Work out the finished part from the listing and answer in its coordinate system (mm). Coordinates: 2 decimals unless noted, no trailing zeros. Order: outer loops, then holes, each group sorted by start corner. A loop starts at its lowest first (then second) coordinate and runs counter-clockwise, first axis right, second up. Notation, with made-up numbers: M 65,-31 L 78,-31 A12 ccw 78,-17 Z; hole C 54.5,15.5 d5. An arc over 180 degrees is marked long. Write item = value, one per line. Start each with the question number.
Q1. Determine the mould class of faces 1 (the cylindrical face through (-43.24, -3.81, 0.81)), 2 (the flat face through (-6, -34.374, 1)), 3 (the flat face through (35.7, -17, 1)) for opening direction Y: released by +Y, released by -Y, zero draft, split by the parting line, or undercut.
Q2. This flat-tipped pin is pushed along its axis until it touches: P1, Ø1.8, axis at x = -42.05, y = -2.9, coming from the +Z side. Where does it stop, or does it pass through?
Q3. Straight lines are drawn through the part: line 1 along Y through (x, z) = (31.65, 0.5); line 2 along Y through (x, z) = (-5.2, 0.6); line 3 along X through (y, z) = (-3.7, 1). For each, find the intervals that lie inside material, in ascending order.
Q4. Find section A-A on x = 31.65. Give the vertices of the cut face in (y, z), and give its area (3 significant figures).
Autodesk Inventor part; units mm, degrees
ref_plane "YZ Plane" through (0, 0, 0) normal (1, 0, 0) x (0, 1, 0)
ref_plane "XZ Plane" through (0, 0, 0) normal (0, 1, 0) x (-1, 0, 0)
ref_plane "XY Plane" through (0, 0, 0) normal (0, 0, 1) x (1, 0, 0)
sketch "Szkic1" plane through (0, 0, 0) normal (0, 0, 1) x (1, 0, 0)
  circle A0 centre (-5.2, -2.45) radius 1.5
  line L0 (-10.4, 2.5) -> (0, 2.5)
  line L1 (-10.4, 2.5) -> (-10.4, -7.4)
  line L2 (-10.4, -7.4) -> (0, -7.4)
  line L3 (0, 2.5) -> (0, -7.4)
  line L4 (-47.2, 2.5) -> (36.8, 2.5)
  line L5 (-47.2, -36.8743) -> (-47.2, 14.8735)
  line L6 (36.8, -36.8743) -> (36.8, 14.8735)
  line L7 (-47.2, 2.5) -> (36.8, 2.5)
  line L8 (36.8, 2.5) -> (36.8, -36.8743)
  line L9 (36.8, -36.8743) -> (-47.2, -36.8743)
  line L10 (-47.2, -36.8743) -> (-47.2, 2.5)
  line L11 (-44.7, -34.3743) -> (34.3, -34.3743)
  line L12 (34.3, -34.3743) -> (34.3, 0)
  line L13 (34.3, 0) -> (-44.7, 0)
  line L14 (-44.7, 0) -> (-44.7, -34.3743)
  line L15 (-5.2, 0) -> (-5.2, -7.4)
  circle A1 centre (-5.2, -3.7) radius 1.5
  point P0 (0, 0)
  dimension "d0" = 2.5
extrude "Wyciągnięcie proste1" add sketch "Szkic1" along normal blind 1.6 contours A0 A1 L15 | A0 L15 L13 L3 L2 A1 | L15 A1 A0 | A0 A1 L15 L2 L1 L13 | L13 L12 L11 L14 L1 L2 L3 picked at (-4.9756, -1.8088) picked at (-5.4233, -1.8086)
sketch "Szkic2" plane through (0, 0, 1.6) normal (0, 0, 1) x (1, 0, 0)
  circle A0 centre (-42.05, -2.9) radius 1.5
  circle A1 centre (31.65, -2.9) radius 1.5
  point P0 (0, 0)
extrude "Wyciągnięcie proste2" cut sketch "Szkic2" against normal through all
sketch "Szkic3" plane through (0, 0, 1.6) normal (0, 0, 1) x (1, 0, 0)
  circle A0 centre (31.65, -2.9) radius 1.5
  circle A1 centre (-42.05, -2.9) radius 1.5
  line L0 (-44.7, 0) -> (-44.7, -34.3743)
  line L1 (-44.7, -34.3743) -> (34.3, -34.3743)
  line L2 (34.3, -34.3743) -> (34.3, 0)
  line L3 (34.3, 0) -> (-44.7, 0)
  circle A2 centre (-5.2, -3.7) radius 1.5
  line L4 (-44.7, 0) -> (-44.7, -34.3743)
  line L5 (34.3, 0) -> (-44.7, 0)
  line L6 (-44.7, -34.3743) -> (34.3, -34.3743)
  line L7 (34.3, -34.3743) -> (34.3, 0)
  line L8 (34.3, 0) -> (-44.7, 0)
  line L9 (-44.7, 0) -> (-44.7, -34.3743)
  line L10 (-46.1, 0) -> (-46.1, -34.3743)
  line L11 (35.7, 0) -> (35.7, -35.7743)
  line L12 (35.7, -35.7743) -> (-44.7, -35.7743)
  line L13 (-46.1, -34.3743) -> (35.7, -34.3743)
  line L14 (-44.7, -34.3743) -> (34.3, -34.3743)
  line L15 (-46.1, 0) -> (35.7, 0)
  point P0 (0, 0)
  dimension "d5" = 1.4
  dimension "d6" = 1.4
extrude "Wyciągnięcie proste3" add sketch "Szkic3" against normal up to surface (1.6 mm away) contours L0 L13 L10 L15 | L15 L11 L13 L2
sketch "Szkic5" plane through (0, 0, 1.6) normal (0, 0, 1) x (1, 0, 0)
  circle A0 centre (31.65, -2.9) radius 1.5
  circle A1 centre (-42.05, -2.9) radius 1.5
  line L0 (-46.1, -34.3743) -> (35.7, -34.3743)
  line L1 (35.7, -34.3743) -> (35.7, 0)
  line L2 (35.7, 0) -> (-46.1, 0)
  line L3 (-46.1, 0) -> (-46.1, -34.3743)
  circle A2 centre (-5.2, -3.7) radius 1.5
  point P0 (0, 0)
properties part number "PCBE_2_2"
Findings below:
q1.face_1 = undercut
q1.face_2 = released by -Y
q1.face_3 = zero draft
q2.P1 = through
q3.line_1 = -34.37 to -4.4, -1.4 to 0
q3.line_2 = -34.37 to -5.2, -2.2 to 0
q3.line_3 = -46.1 to -43.32, -40.78 to -6.7, -3.7 to 30.38, 32.92 to 35.7
q4.outline = M -34.37,0 L -4.4,0 L -4.4,1.6 L -34.37,1.6 Z; M -1.4,0 L 0,0 L 0,1.6 L -1.4,1.6 Z
q4.area = 50.2 mm^2
